Could you check a few things on this model? Use its own coordinates, in mm. A direction names the side the tool comes from. Coordinates: 2 decimals unless noted, no trailing zeros. Loops run counter-clockwise (first coordinate to the right, second up) from the corner with the lowest first, then second, coordinate; pieces in that order, holes last. Notation, with made-up numbers: (16.5, 87) - (51.5, 87) arc R18 cw to (51.5, 111) - close; hole circle Ø4 at (41, 71). An arc over 180 degrees is marked (long way). One line per question, with ' | ' between items. Start each with the question number.
1. Please list where these lines run through material, in increasing order: L1, parallel to X at y = 1, z = 3; L2, parallel to Y at x = -43.5, z = 7; L3, parallel to Z at x = 9, y = -28.5. Write a range as [from, to].
2. I want a section at A-A, the plane z = 2. Write out the boundary of the cut face in (x, y).
3. We'd pull the mould along Z, two halves only. Please class faces 3 (the flat face through (2.491, 9.826, 25.808)), 4 (the cylindrical face through (62.417, 12.466, 13.551)), 5 (the cylindrical face through (62.417, -9.495, -2.248)): pulls with the +Z half, pulls with the -Z half, needs draft (parallel to the pull), parting line crosses it, or undercut.
4. I want a section at C-C, the plane x = -52. Write out the boundary of the cut face in (y, z), then the cut area to 3 significant figures.
5. Which directions (+Z, -Z, +X, -X, +Y, -Y) give clear straight access to the entire face, cutting with the end or side of a thin tool? Please do faces 1 (the flat face through (-1, 9.218, 12)), 2 (the flat face through (-1, -9, -3)).
6. I'm going to push a flat-ended pin straight in: P1, Ø12, axis at x = 31, y = -21, coming from the +Z side. Where does the tip first touch, or does it pass through?
7. I want a section at B-B, the plane y = 4.5. Write out the boundary of the cut face in (x, z), then the cut area to 3 significant figures.
from build123d import *

# Parameters (mm, degrees)
F0_W     = 126
F0_H     = 46
F0_W_2   = 120
F0_H_2   = 38
F1_DEPTH = 3
F2_DEPTH = 28
F4_DEPTH = 123
F5_R     = 2.5


with BuildPart() as f1:
    # F0 (on Top) → F1 (new body)
    with BuildSketch(Plane.XY):
        with Locations((0.13021, -9.781944)):
            Rectangle(F0_W, F0_H)
        with Locations((0.13021, -9.781944)):
            Rectangle(F0_W_2, F0_H_2, mode=Mode.SUBTRACT)
        with Locations((0.13021, -9.781944)):
            Rectangle(F0_W_2, F0_H_2)
    extrude(amount=-F1_DEPTH)

    # F0 (on Top) → F2 (join)
    with BuildSketch(Plane.XY):
        with Locations((0.13021, -9.781944)):
            Rectangle(F0_W, F0_H)
        with Locations((0.13021, -9.781944)):
            Rectangle(F0_W_2, F0_H_2, mode=Mode.SUBTRACT)
    extrude(amount=F2_DEPTH)

    # F3 (on face) → F4 (cut)
    with BuildSketch(Plane.YZ.offset(63.13021)):
        Polygon((9.218056, 28), (-28.781944, 28), (-29.981944, 23.676099), (-28.781944, 23.676099), (9.218056, 23.676099), (10.418056, 23.676099), align=None)
    extrude(amount=-F4_DEPTH, mode=Mode.SUBTRACT)

    # F5
    f5_edges = [f1.edges().sort_by_distance(p)[0] for p in [
        (63.13021, -32.781944, 12.5),
        (63.13021, 13.218056, 12.5),
        (-62.86979, -32.781944, 12.5),
        (-62.86979, 13.218056, 12.5),
        (0.13021, 13.218056, -3),
        (63.13021, -9.781944, -3),
        (0.13021, -32.781944, -3),
        (-62.86979, -9.781944, -3),
        (0.13021, -32.781944, 28),
        (-62.86979, -9.781944, 28),
        (0.13021, 13.218056, 28),
    ]]
    fillet(f5_edges, radius=F5_R)


solid = f1.part
Results are:
1) L1: x = [-62.87, -59.87], [60.13, 63.13] | L2: y = [-32.78, -28.78], [9.22, 13.22] | L3: z = [-3, 0]
2) outline: (-62.87, -30.28) arc R2.5 ccw to (-60.37, -32.78) - (60.63, -32.78) arc R2.5 ccw to (63.13, -30.28) - (63.13, 10.72) arc R2.5 ccw to (60.63, 13.22) - (-60.37, 13.22) arc R2.5 ccw to (-62.87, 10.72) - close; hole (-59.87, -28.78) - (60.13, -28.78) - (60.13, 9.22) - (-59.87, 9.22) - close
3) face 3: undercut | face 4: needs draft | face 5: pulls with the -Z half
4) outline: (-32.78, -0.5) arc R2.5 ccw to (-30.28, -3) - (10.72, -3) arc R2.5 ccw to (13.22, -0.5) - (13.22, 25.5) arc R2.5 ccw to (10.72, 28) - (9.22, 28) - (10.42, 23.68) - (9.22, 23.68) - (9.22, 0) - (-28.78, 0) - (-28.78, 23.68) - (-29.98, 23.68) - (-28.78, 28) - (-30.28, 28) arc R2.5 ccw to (-32.78, 25.5) - close | area: 351 mm2
5) face 1: +Z | face 2: -Z, +X, -X, +Y, -Y
6) P1: stops at z = 0
7) outline: (-62.87, -0.5) arc R2.5 ccw to (-60.37, -3) - (60.63, -3) arc R2.5 ccw to (63.13, -0.5) - (63.13, 23.68) - (60.13, 23.68) - (60.13, 0) - (-59.87, 0) - (-59.87, 28) - (-60.37, 28) arc R2.5 ccw to (-62.87, 25.5) - close | area: 529 mm2
